```python
from build123d import *

# Parameters (mm, degrees)
SKETCH1_W             = 5
SKETCH1_H             = 63.5
BOSS_EXTRUDE1_DEPTH   = 65
BOSS_EXTRUDE1_2_DEPTH = 65
SKETCH1_4_R           = 72.5
BOSS_EXTRUDE2_DEPTH   = 7
BOSS_EXTRUDE3_DEPTH   = 5
BOSS_EXTRUDE4_START   = -5
BOSS_EXTRUDE4_DEPTH   = 5
SKETCH4_R             = 30
BOSS_EXTRUDE5_DEPTH   = 7
SKETCH5_R             = 32
BOSS_EXTRUDE6_DEPTH   = 2
SKETCH6_R             = 10
BOSS_EXTRUDE7_DEPTH   = 17
SKETCH13_R            = 3.5
SKETCH13_R_2          = 2
CUT_EXTRUDE3_DEPTH    = 5
SKETCH14_R            = 10
CUT_EXTRUDE4_DEPTH    = 5


with BuildPart() as part:
    # Sketch1 → Boss-Extrude1 (new body)
    with BuildSketch(Plane.XY):
        with Locations((58.75, 0)):
            Rectangle(SKETCH1_W, SKETCH1_H)
    extrude(amount=BOSS_EXTRUDE1_DEPTH)



with BuildPart() as body_2:
    # Sketch1 → Boss-Extrude1 2 (new body)
    with BuildSketch(Plane.XY):
        with Locations((-58.75, 0)):
            Rectangle(SKETCH1_W, SKETCH1_H)
    extrude(amount=BOSS_EXTRUDE1_2_DEPTH)


with BuildPart() as part_1:
    add(part.part)

    add(body_2.part)  # Boss-Extrude2 merges body 2
    # Sketch1<4> → Boss-Extrude2 (add)
    with BuildSketch(Plane.XY):
        Circle(SKETCH1_4_R)
    extrude(amount=-BOSS_EXTRUDE2_DEPTH)

    # Sketch2 → Boss-Extrude3 (add)
    with BuildSketch(Plane.ZY.offset(-56.25)):
        with BuildLine():
            Line((65, -31.75), (65, 31.75))
            ThreePointArc((65, 31.75), (96.75, 0), (65, -31.75))
        make_face()
    extrude(amount=-BOSS_EXTRUDE3_DEPTH)

    # Sketch3 → Boss-Extrude4 (add)
    with BuildSketch(Plane(origin=(-56.25, 0, 0), x_dir=(0, 0, -1), z_dir=(1, 0, 0)).offset(BOSS_EXTRUDE4_START)):
        with BuildLine():
            Line((-65, 31.75), (-65, -31.75))
            ThreePointArc((-65, -31.75), (-96.75, 0), (-65, 31.75))
        make_face()
    extrude(amount=BOSS_EXTRUDE4_DEPTH)

    # Sketch4 → Boss-Extrude5 (add)
    with BuildSketch(Plane(origin=(0, 0, -7), x_dir=(-1, 0, 0), z_dir=(0, 0, -1))):
        Circle(SKETCH4_R)
    extrude(amount=BOSS_EXTRUDE5_DEPTH)

    # Sketch5 → Boss-Extrude6 (add)
    with BuildSketch(Plane(origin=(0, 0, -14), x_dir=(-1, 0, 0), z_dir=(0, 0, -1))):
        Circle(SKETCH5_R)
    extrude(amount=BOSS_EXTRUDE6_DEPTH)

    # Sketch6 → Boss-Extrude7 (add)
    with BuildSketch(Plane(origin=(0, 0, -16), x_dir=(-1, 0, 0), z_dir=(0, 0, -1))):
        Circle(SKETCH6_R)
    extrude(amount=BOSS_EXTRUDE7_DEPTH)

    # Sketch13 → Cut-Extrude3 (cut)
    with BuildSketch(Plane(origin=(61.25, 0, 0), x_dir=(0, 0, -1), z_dir=(1, 0, 0))):
        with Locations((-66.505993966, 0)):
            Circle(SKETCH13_R)
        with Locations((-76.505993966, 0)):
            Circle(SKETCH13_R_2)
        with Locations((-66.505993966, -10)):
            Circle(SKETCH13_R_2)
        with Locations((-56.505993966, 0)):
            Circle(SKETCH13_R_2)
        with Locations((-66.505993966, 10)):
            Circle(SKETCH13_R_2)
    extrude(amount=-CUT_EXTRUDE3_DEPTH, mode=Mode.SUBTRACT)

    # Sketch14 → Cut-Extrude4 (cut)
    with BuildSketch(Plane.ZY.offset(61.25)):
        with Locations((65.530908604, 0)):
            Circle(SKETCH14_R)
    extrude(amount=-CUT_EXTRUDE4_DEPTH, mode=Mode.SUBTRACT)


solid = part_1.part
```
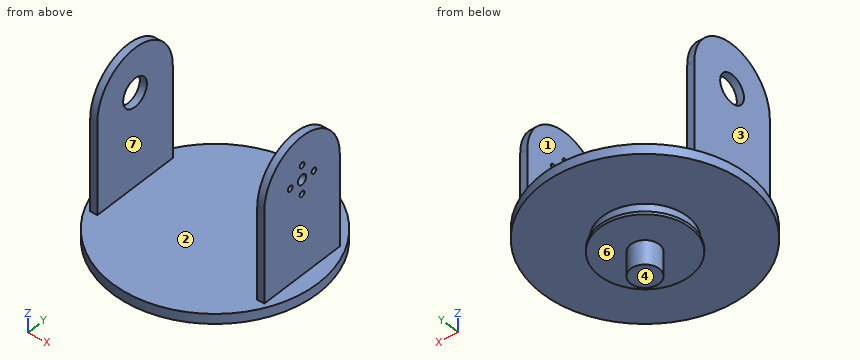
Verification items for the finished model (mm, model axes). Face numbers are marked on the shaded views. A direction names the side the tool comes from. Round coordinates to 2 decimals unless told otherwise and drop trailing zeros. Write each loop counter-clockwise with the first axis right and the second up, starting at its lowest first coordinate (ties: lowest second). Pieces come first, ordered by that corner, then holes.
1. Draft check along X on the marked faces 1, 2, 3 and 4. Enter one of: +X half, -X half, draft (parallel to the pull), parting line (faces both ways), or undercut.
2. Section check D-D on y = -52.5. Enter the section's corners in (x, z), plus the area to 3 significant figures.
3. Section check A-A on z = 33. Enter the section's corners in (x, y), plus the area to 3 significant figures.
4. Section check C-C on y = 0. State how many separate pieces and enclosed holes the cut face has, plus the area to 3 significant figures.
5. Access from +Z, -Z, +X, -X, +Y, -Y to the whole of each face (thin tool, end or side, straight path). Record for the marked faces 5, 6 and 7.
6. Section check B-B on x = 0. Enter the section's corners in (y, z), plus the area to 3 significant figures.
7. Scan lines: L1, parallel to X at y = 20, z = 46.5; L2, parallel to Z at x = -63.5, y = 26; L3, parallel to X at y = 0.5, z = -2. Record each from-to range of solid material in increasing order.
8. Gauge pin test, flat ends, axial feed: P1, Ø16, axis at y = 0, z = 65.53, coming from the -X side; P2, Ø5, axis at x = 12.5, y = 50, coming from the +Z side; P3, Ø3, axis at y = 10, z = 66.51, coming from the -X side. Record the tip position at first contact, or that the pin passes through.
Answer:
1. face 1: undercut
1. face 2: undercut
1. face 3: -X half
1. face 4: draft
2. outline: (-50, -7) - (50, -7) - (50, 0) - (-50, 0) - close
2. area: 700 mm2
3. outline: (-61.25, -31.75) - (-56.25, -31.75) - (-56.25, 31.75) - (-61.25, 31.75) - close; (56.25, -31.75) - (61.25, -31.75) - (61.25, 31.75) - (56.25, 31.75) - close
3. area: 635 mm2
4. separate pieces: 5
4. enclosed holes: 0
4. area: 2,700 mm2
5. face 5: +Z, +X, +Y, -Y
5. face 6: -Z
5. face 7: +Z, +Y, -Y
6. outline: (-72.5, -7) - (-30, -7) - (-30, -14) - (-32, -14) - (-32, -16) - (-10, -16) - (-10, -33) - (10, -33) - (10, -16) - (32, -16) - (32, -14) - (30, -14) - (30, -7) - (72.5, -7) - (72.5, 0) - (-72.5, 0) - close
6. area: 1,900 mm2
7. L1: x = -61.25 to -56.25, 56.25 to 61.25
7. L2: z = -7 to 0
7. L3: x = -72.5 to 72.5
8. P1: stops at x = 56.25
8. P2: stops at z = 0
8. P3: stops at x = -61.25
